Geometry: final body of the model. Coordinates: model frame, mm. A direction names the side the tool comes from. Coordinates: 2 decimals unless noted, no trailing zeros. Order: outer loops, then holes, each group sorted by start corner. A loop starts at its lowest first (then second) coordinate and runs counter-clockwise, first axis right, second up. Notation, with made-up numbers: M 63,43.25 L 107,43.25 A31 cw 107,71.25 Z; hole C 40.25,57.5 d8. An arc over 180 degrees is marked long. Use CSV: the item, a comma, the result in double quotes. Start each with the question number.
Q1. Mould query, pull axis Z, two halves, no side actions, for faces 3 (the face through (17, 0.816, -19)), 4 (the face through (-8, 0, -21)), 5 (the face through (-25.865, 1.479, 10.724)). Classes: +Z half, -Z half, draft (parallel to the pull), parting line (faces both ways), or undercut.
Q2. First-contact query: P1, Ø5.5, axis at x = 18.025, z = -18.025, coming from the +Y side; P2, Ø1.4, axis at x = 19, z = -17, coming from the +Y side; P3, Ø1, axis at y = 0.5, z = -1.5, coming from the +X side; P4, Ø1, axis at x = 0.5, y = 2.5, coming from the +Z side. Flat tips, straight axial feed; report the tip coordinate or a pass-through.
Q3. Section query B-B, the plane x = 0. Output: boundary loops of the cut face in (y, z).
Q4. Section query C-C, the plane y = 2.5. Output: boundary loops of the cut face in (x, z) (1 decimal).
Q5. Access query for faces 1 (the face through (-18.935, 1.893, -19.78)), 2 (the face through (-18.353, 0.402, -17.37)). Directions: +Z, -Z, +X, -X, +Y, -Y. A direction counts if a zero-diameter tool reaches every point of the face in a straight line with its end or side. Return the directions, or none.
Q6. Section query A-A, the plane z = 0. Output: boundary loops of the cut face in (x, y), and give its area (3 significant figures).
Q7. Ray query, probe 1 along Z at (x, y) = (19, 2); probe 2 along Z at (x, y) = (-16.5, 2); probe 3 along Z at (x, y) = (-5, 0.7). Return the intervals inside material, ascending.
Q8. Section query D-D, the plane z = 23.5. Output: boundary loops of the cut face in (x, y).
Autodesk Inventor part; units mm, degrees
ref_plane "YZ Plane" through (0, 0, 0) normal (1, 0, 0) x (0, 1, 0)
ref_plane "XZ Plane" through (0, 0, 0) normal (0, 1, 0) x (-1, 0, 0)
ref_plane "XY Plane" through (0, 0, 0) normal (0, 0, 1) x (1, 0, 0)
sketch "Sketch1" plane through (0, 0, 0) normal (0, 1, 0) x (-1, 0, 0)
  circle A0 centre (0, 0) radius 22
  circle A1 centre (0, 0) radius 28
  dimension "d0" = 44
  dimension "d1" = 56
extrude "Extrusion1" add sketch "Sketch1" along normal blind 3
sketch "Sketch5" plane through (0, 3, 0) normal (0, 1, 0) x (1, 0, 0)
  line L0 (18.025, 18.025) -> (-17.325, 18.025)
  line L1 (-17.325, 18.025) -> (-17.325, -17.325)
  line L2 (-17.325, -17.325) -> (18.025, -17.325)
  line L3 (18.025, -17.325) -> (18.025, 18.025)
  point P0 (0, 0)
  dimension "d22" = 35.35
  dimension "d23" = 35.35
hole "Hole3" at (-17.325, 3, 17.325) at (-17.325, 3, -18.025) at (18.025, 3, -18.025) at (18.025, 3, 17.325) direction (0, -1, 0) diameter 2.438 end through all counterbore diameter 4.763 counterbore depth 2.184
properties part number "chamberPlateCircle"
Responses:
1,face 3,"undercut"
1,face 4,"draft"
1,face 5,"parting line"
2,P1,"stops at y = 3"
2,P2,"stops at y = 0.82"
2,P3,"stops at x = 27.98"
2,P4,"stops at z = 28"
3,outline,"M 0,-28 L 3,-28 L 3,-22 L 0,-22 Z; M 0,22 L 3,22 L 3,28 L 0,28 Z"
4,outline,"C 0,0 d56; hole C 0,0 d44; hole C -17.3,-18 d4.8; hole C -17.3,17.3 d4.8; hole C 18,-18 d4.8; hole C 18,17.3 d4.8"
5,face 1,"+Y"
5,face 2,"+Y, -Y"
6,outline,"M -28,0 L -22,0 L -22,3 L -28,3 Z; M 22,0 L 28,0 L 28,3 L 22,3 Z"
6,area,"36.0 mm²"
7,probe 1,"z = -20.57 to -20.2, -15.85 to -11.09, 11.09 to 15.15, 19.5 to 20.57"
7,probe 2,"z = -22.62 to -20.26, -15.79 to -14.55, 14.55 to 15.09, 19.56 to 22.62"
7,probe 3,"z = -27.55 to -21.42, 21.42 to 27.55"
8,outline,"M -15.22,0 L 15.22,0 L 15.22,3 L -15.22,3 Z"
